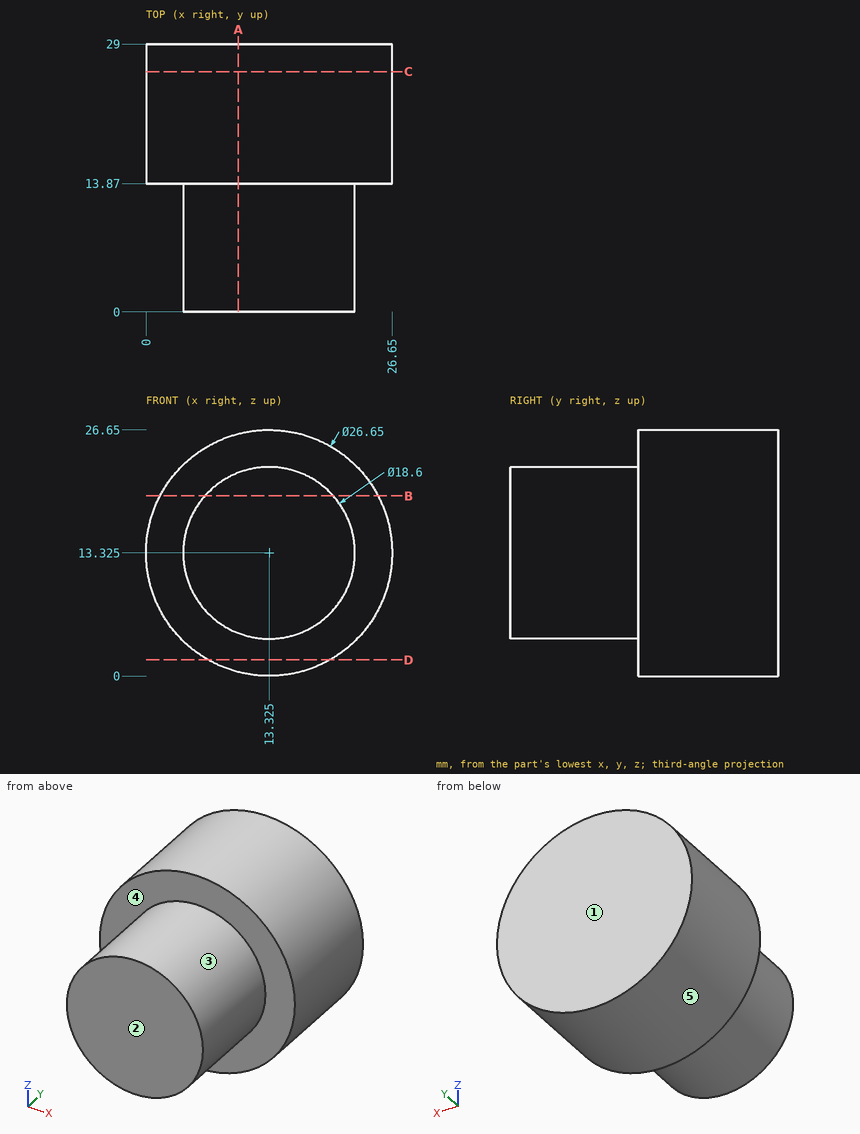
Can you work these out from the drawing? Everything is in mm from the part's minimum corner. A direction names the side the tool comes from. Round coordinates to 2 decimals unless told otherwise and drop trailing zeros. Order: outer loops, then holes, each group sorted by start corner. A loop starts at its lowest first (then second) coordinate and runs counter-clockwise, first axis right, second up. Notation, with made-up numbers: (50.5, -12.75) -> (96.5, -12.75) arc R8 cw to (96.5, -4.75) -> close; hole circle Ø10 at (4.5, -38). An arc over 180 degrees is marked (long way). Return JSON: item names as keys, results as strings. Group by question number.
1. Will these pins go through, and if not, where does the flat tip stop? pin 1 (1.5 mm diameter, centred on y = 22, z = 18.5, fed in from +X); pin 2 (1.5 mm diameter, centred on y = 9.5, z = 14, fed in from +X) (3 decimals); pin 3 (8 mm diameter, centred on x = 4, y = 18, fed in from -Z).
2. We'd pull the mould along Y, two halves only. Please class the marked faces 1, 2 and 3: released by +Y, released by -Y, zero draft, split by the parting line, or undercut.
3. Which directions (+Z, -Z, +X, -X, +Y, -Y) give clear straight access to the entire face, cutting with the end or side of a thin tool? Please do the marked faces 4 and 5.
4. I need wall thicknesses on line 1 (Y direction, x = 2.75, z = 7); line 2 (X direction, y = 24.5, z = 13); line 3 (Z direction, x = 23, y = 26.5). Which ranges of each line are inside material? Lowest first, please. Write a range as [from, to].
5. If we section it at D-D, the plane z = 1.75: Write out the boundary of the cut face in (x, y), then the cut area to 3 significant figures.
6. If we section it at B-B, the plane z = 19.5: Write out the boundary of the cut face in (x, y).
7. If we section it at A-A, the plane x = 10: Write out the boundary of the cut face in (y, z).
8. If we section it at C-C, the plane y = 26: Write out the boundary of the cut face in (x, z) (3 decimals), then the cut area to 3 significant figures.
Output values:
{
 "1": {"pin 1": "x = 25.89", "pin 2": "x = 22.625", "pin 3": "z = 1.11"},
 "2": {"face 1": "released by +Y", "face 2": "released by -Y", "face 3": "zero draft"},
 "3": {"face 4": "-Y", "face 5": "+Y, -Y"},
 "4": {"line 1": "[13.87, 29]", "line 2": "[0, 26.65]", "line 3": "[4.16, 22.49]"},
 "5": {"outline": "(6.72, 13.87) -> (19.93, 13.87) -> (19.93, 29) -> (6.72, 29) -> close", "area": "200 mm²"},
 "6": {"outline": "(1.52, 13.87) -> (6.37, 13.87) -> (6.37, 0) -> (20.28, 0) -> (20.28, 13.87) -> (25.13, 13.87) -> (25.13, 29) -> (1.52, 29) -> close"},
 "7": {"outline": "(0, 4.64) -> (13.87, 4.64) -> (13.87, 0.42) -> (29, 0.42) -> (29, 26.23) -> (13.87, 26.23) -> (13.87, 22.01) -> (0, 22.01) -> close"},
 "8": {"outline": "circle Ø26.65 at (13.325, 13.325)", "area": "558 mm²"}
}
